```python
from build123d import *

# Parameters (mm, degrees)
SKETCH1_W           = 12.6
SKETCH1_H           = 19
BOSS_EXTRUDE1_DEPTH = 8
CUT_EXTRUDE1_DEPTH  = 20
CUT_EXTRUDE2_DEPTH  = 13.6
SKETCH4_R           = 0.675
CUT_EXTRUDE3_DEPTH  = 0.3
SKETCH5_R           = 0.3
BOSS_EXTRUDE2_DEPTH = 3.55


with BuildPart() as part:
    # Sketch1 → Boss-Extrude1 (new body)
    with BuildSketch(Plane(origin=(0, 0, 0), x_dir=(1, 0, 0), z_dir=(0, 1, 0))):
        Rectangle(SKETCH1_W, SKETCH1_H)
    extrude(amount=BOSS_EXTRUDE1_DEPTH)

    # Sketch2 → Cut-Extrude1 (cut, through all)
    with BuildSketch(Plane.XY.offset(9.5)):
        Polygon((-4.92, 0), (4.92, 0), (4.42, 1), (-4.42, 1), align=None)
    extrude(amount=-CUT_EXTRUDE1_DEPTH, mode=Mode.SUBTRACT)

    # Sketch3 → Cut-Extrude2 (cut, through all)
    with BuildSketch(Plane.ZY.offset(6.3)):
        Polygon((-7.62, 0), (7.62, 0), (7.12, 1), (-7.12, 1), align=None)
    extrude(amount=-CUT_EXTRUDE2_DEPTH, mode=Mode.SUBTRACT)

    # Sketch4 → Cut-Extrude3 (cut)
    with BuildSketch(Plane(origin=(0, 8, 0), x_dir=(1, 0, 0), z_dir=(0, 1, 0))):
        with Locations((4.8, -6.39)):
            Circle(SKETCH4_R)
        Polygon((-1.408090595, 7.057802146), (3.391909405, 7.057802146), (3.204025719, 5.720940254), (-1.595974281, 5.720940254), align=None)
        Polygon((-3.198514004, -5.681722368), (1.601485996, -5.681722368), (1.396229552, -7.142197854), (-3.403770448, -7.142197854), align=None)
        Polygon((-3.048549266, 0), (-2.373549266, 0.675), (2.373549266, 0.675), (3.048549266, 0), (2.373549266, -0.675), (-2.373549266, -0.675), align=None)
        with BuildLine():
            Line((3.694857677, 7.057802146), (2.797813335, 0.675))
            Line((2.797813335, 0.675), (3.322813335, 0.15))
            Line((3.322813335, 0.15), (4.08729662, 0.15))
            Line((4.08729662, 0.15), (4.930044629, 6.146463666))
            ThreePointArc((4.930044629, 6.146463666), (4.741597838, 6.78264937), (4.137830174, 7.057802146))
            Line((4.137830174, 7.057802146), (3.694857677, 7.057802146))
        make_face()
        with BuildLine():
            Line((3.339208356, -0.15), (4.094226883, -0.15))
            Line((4.094226883, -0.15), (3.208322625, -6.453536334))
            ThreePointArc((3.208322625, -6.453536334), (2.940955393, -6.945965518), (2.41610817, -7.142197854))
            Line((2.41610817, -7.142197854), (1.748270337, -7.142197854))
            Line((1.748270337, -7.142197854), (2.631497367, -0.857710989))
            Line((2.631497367, -0.857710989), (3.339208356, -0.15))
        make_face()
        with BuildLine():
            Line((-1.711038867, 7.057802146), (-2.577058081, 0.895755255))
            Line((-2.577058081, 0.895755255), (-3.322813335, 0.15))
            Line((-3.322813335, 0.15), (-4.045134369, 0.15))
            Line((-4.045134369, 0.15), (-3.171091155, 6.369140627))
            ThreePointArc((-3.171091155, 6.369140627), (-2.903723923, 6.861569811), (-2.3788767, 7.057802146))
            Line((-2.3788767, 7.057802146), (-1.711038867, 7.057802146))
        make_face()
        with BuildLine():
            Line((-4.08729662, -0.15), (-4.941905672, -6.230859373))
            ThreePointArc((-4.941905672, -6.230859373), (-4.753458881, -6.867045077), (-4.149691217, -7.142197854))
            Line((-4.149691217, -7.142197854), (-3.70671872, -7.142197854))
            Line((-3.70671872, -7.142197854), (-2.797813335, -0.675))
            Line((-2.797813335, -0.675), (-3.322813335, -0.15))
            Line((-3.322813335, -0.15), (-4.08729662, -0.15))
        make_face()
    extrude(amount=-CUT_EXTRUDE3_DEPTH, mode=Mode.SUBTRACT)

    # Sketch5 → Boss-Extrude2 (add)
    with BuildSketch(Plane.XZ.offset(-1)):
        with Locations((-4.92, 7.62)):
            Circle(SKETCH5_R)
        with Locations((-2.46, 7.62)):
            Circle(SKETCH5_R)
        with Locations((0, 7.62)):
            Circle(SKETCH5_R)
        with Locations((2.46, 7.62)):
            Circle(SKETCH5_R)
        with Locations((4.92, 7.62)):
            Circle(SKETCH5_R)
        with Locations((-2.46, -7.62)):
            Circle(SKETCH5_R)
        with Locations((0, -7.62)):
            Circle(SKETCH5_R)
        with Locations((2.46, -7.62)):
            Circle(SKETCH5_R)
        with Locations((4.92, -7.62)):
            Circle(SKETCH5_R)
        with Locations((-4.92, -7.62)):
            Circle(SKETCH5_R)
    extrude(amount=BOSS_EXTRUDE2_DEPTH)


solid = part.part
```
Here's how the part is built. I have some questions about the finished solid (model axes, mm). A direction names the side the tool comes from. Round coordinates to 2 decimals unless told otherwise and drop trailing zeros. Order: outer loops, then holes, each group sorted by start corner. A loop starts at its lowest first (then second) coordinate and runs counter-clockwise, first axis right, second up. Notation, with made-up numbers: M -18,31 L 33,31 A15 cw 33,53 Z; hole C 21,-25 d8. An arc over 180 degrees is marked long. Answer in a Markdown table with one row per item.
Item 1: Thinking about a two-plate mould opening in X: for faces 1 (the face through (0, 4, 9.5)), 2 (the face through (-6.3, 4, 0)), 3 (the face through (4.674, 0.493, 8.591)), which applies, +X half, -X half, draft (parallel to the pull), parting line (faces both ways), or undercut?
A:
| item | result |
|---|---|
| face 1 | draft |
| face 2 | -X half |
| face 3 | undercut |
Item 2: If I drill on L1, parallel to X at y = 7.9, z = 6.39 (3 decimals); L2, parallel to Y at x = -1, z = -5.5; L3, parallel to Y at x = 3.5, z = -3.25, over which ranges is the centre line in solid material (lowest first)? Write a range as from..to.
A:
| item | result |
|---|---|
| L1 | x = -6.3..-4.948, -3.601..-3.298, 1.502..1.854, 3.217..4.125, 5.475..6.3 |
| L2 | y = 1..8 |
| L3 | y = 1..7.7 |
Item 3: Imagine slicing it at A-A, the plane y = -1.5. State how many separate pieces and enclosed holes the cut face has, and give its area (3 significant figures).
A:
| item | result |
|---|---|
| separate pieces | 10 |
| enclosed holes | 0 |
| area | 2.83 mm2 |
Item 4: Imagine slicing it at C-C, the plane z = -1.25. Write out the boundary of the cut face in (x, y).
A:
| item | result |
|---|---|
| outline | M -6.3,1 L 6.3,1 L 6.3,8 L 4.24,8 L 4.24,7.7 L 2.88,7.7 L 2.88,8 L -2.53,8 L -2.53,7.7 L -3.89,7.7 L -3.89,8 L -6.3,8 Z |
Item 5: I'm going to push flat-ended pins straight in: pin 1 (2 mm diameter, centred on x = -3.5, z = 6, fed in from -Y); pin 2 (1.5 mm diameter, centred on x = -6, z = 8.5, fed in from -Y); pin 3 (0.7 mm diameter, centred on x = 1, z = -6.5, fed in from +Y). Where does each tip first touch, or does it pass through?
A:
| item | result |
|---|---|
| pin 1 | stops at y = 1 |
| pin 2 | stops at y = 0 |
| pin 3 | stops at y = 7.7 |
Item 6: Imagine slicing it at B-B, the plane x = -0.75. Write out the boundary of the cut face in (y, z) (3 decimals), and give its area (3 significant figures).
A:
| item | result |
|---|---|
| outline | M 1,-9.5 L 8,-9.5 L 8,-7.058 L 7.7,-7.058 L 7.7,-5.721 L 8,-5.721 L 8,-0.675 L 7.7,-0.675 L 7.7,0.675 L 8,0.675 L 8,5.682 L 7.7,5.682 L 7.7,7.142 L 8,7.142 L 8,9.5 L 1,9.5 Z |
| area | 132 mm2 |
Item 7: For faces 4 (the face through (6.3, 4, 0)), 5 (the face through (-3, 7.7, -4)), which set-ups out of +Z, -Z, +X, -X, +Y, -Y let a thin tool reach every point of the face, with its end or its side?
A:
| item | result |
|---|---|
| face 4 | +Z, -Z, +X, +Y, -Y |
| face 5 | +Y |
